Can you work these out from the model? Positions are in its coordinate system, mm. Face numbers are marked on the shaded views. A direction names the side the tool comes from. Coordinates: 2 decimals unless noted, no trailing zeros. Loops run counter-clockwise (first coordinate to the right, second up) from the corner with the lowest first, then second, coordinate; pieces in that order, holes last. Notation, with made-up numbers: M 51.5,84 L 55.5,84 A9 cw 55.5,96 Z; hole C 32.25,67.25 d5. An arc over 180 degrees is marked long. Return JSON: item names as keys, results as strings. Group by question number.
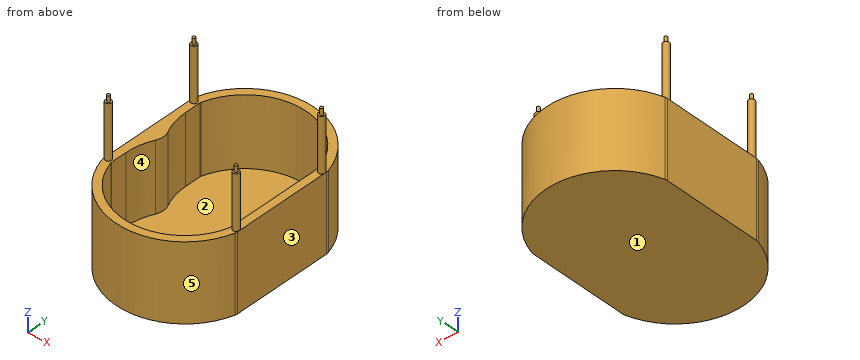
```python
from build123d import *

# Parameters (mm, degrees)
F0_R     = 6
F1_DEPTH = 150
F2_T     = -15
F4_DEPTH = 135
F5_DEPTH = 105
F6_R     = 3
F7_DEPTH = 12


# Not quite as in the source:
# - a feature names something its author has since deleted; it is built from what else it names


with BuildPart() as f1:
    # F0 (on Top) → F1 (new body)
    with BuildSketch(Plane.XY):
        with BuildLine():
            Line((-131, -92.5), (-131, -95.859159479))
            ThreePointArc((-131, -95.859159479), (-130.8132026368, -98.5862460693), (-130.2562998729, -101.2623914012))
            ThreePointArc((-130.2562998729, -101.2623914012), (0, -200), (130.2562998729, -101.2623914012))
            ThreePointArc((130.2562998729, -101.2623914012), (130.8132026368, -98.5862460693), (131, -95.859159479))
            Line((131, -95.859159479), (131, -92.5))
            Line((131, -92.5), (131, 92.5))
            Line((131, 92.5), (131, 95.859159479))
            ThreePointArc((131, 95.859159479), (130.8132026368, 98.5862460693), (130.2562998729, 101.2623914012))
            ThreePointArc((130.2562998729, 101.2623914012), (0, 200), (-130.2562998729, 101.2623914012))
            ThreePointArc((-130.2562998729, 101.2623914012), (-130.8132026368, 98.5862460693), (-131, 95.859159479))
            Line((-131, 95.859159479), (-131, 92.5000001623))
            Line((-131, 92.5000001623), (-131, -92.5))
        make_face()
        with BuildLine():
            ThreePointArc((-119, -92.5), (-125, -98.5), (-131, -92.5))
            ThreePointArc((-131, -92.5), (-125, -86.5), (-119, -92.5))
        make_face(mode=Mode.SUBTRACT)
        with Locations((125, -92.5)):
            Circle(F0_R, mode=Mode.SUBTRACT)
        with BuildLine():
            ThreePointArc((-119, 92.5), (-125.0000000812, 86.5), (-131, 92.5000001623))
            ThreePointArc((-131, 92.5000001623), (-124.9999999188, 98.5), (-119, 92.5))
        make_face(mode=Mode.SUBTRACT)
        with Locations((125, 92.5)):
            Circle(F0_R, mode=Mode.SUBTRACT)
        with BuildLine():
            ThreePointArc((-119, -92.5), (-125, -86.5), (-131, -92.5))
            ThreePointArc((-131, -92.5), (-125, -98.5), (-119, -92.5))
        make_face()
        with BuildLine():
            ThreePointArc((-119, 92.5), (-124.9999999188, 98.5), (-131, 92.5000001623))
            ThreePointArc((-131, 92.5000001623), (-125.0000000812, 86.5), (-119, 92.5))
        make_face()
        with Locations((125, -92.5)):
            Circle(F0_R)
        with Locations((125, 92.5)):
            Circle(F0_R)
    extrude(amount=-F1_DEPTH)

    # F2
    f2_openings = [f1.faces().sort_by_distance(p)[0] for p in [
        (0, 0, 0),
    ]]
    offset(amount=F2_T, openings=f2_openings)

    # F3 (on face) → F4 (join, through all)
    with BuildSketch(Plane.XY):
        with BuildLine():
            ThreePointArc((-103.9827400965, 13.2972029152), (-112.95573879, 38.3122762743), (-116, 64.7130541872))
            Line((-116, 64.7130541872), (-116, -64.7130541872))
            ThreePointArc((-116, -64.7130541872), (-112.95573879, -38.3122762743), (-103.9827400965, -13.2972029152))
            ThreePointArc((-103.9827400965, -13.2972029152), (-100.8748280525, 0), (-103.9827400965, 13.2972029152))
        make_face()
    extrude(amount=-F4_DEPTH)

    # F0 (on Top) → F5 (join)
    with BuildSketch(Plane.XY):
        with Locations((125, -92.5)):
            Circle(F0_R)
        with Locations((125, 92.5)):
            Circle(F0_R)
        with BuildLine():
            ThreePointArc((-119, 92.5), (-124.9999999188, 98.5), (-131, 92.5000001623))
            ThreePointArc((-131, 92.5000001623), (-125.0000000812, 86.5), (-119, 92.5))
        make_face()
        with BuildLine():
            ThreePointArc((-119, -92.5), (-125, -86.5), (-131, -92.5))
            ThreePointArc((-131, -92.5), (-125, -98.5), (-119, -92.5))
        make_face()
    extrude(amount=F5_DEPTH)

    # F6 (on face) → F7 (join)
    with BuildSketch(Plane.XY.offset(105)):
        with Locations((125, -92.5)):
            Circle(F6_R)
        with Locations((-125, -92.5)):
            Circle(F6_R)
        with Locations((125, 92.5)):
            Circle(F6_R)
        with Locations((-125, 92.5)):
            Circle(F6_R)
    extrude(amount=F7_DEPTH)


solid = f1.part
```
1) If we mould it in two halves opening along X, with no side actions, what happens to the marked faces 1, 2 and 3? For each: +X half, -X half, draft (parallel to the pull), parting line (faces both ways), or undercut.
2) For the marked faces 4 and 5, which set-ups out of +Z, -Z, +X, -X, +Y, -Y let a thin tool reach every point of the face, with its end or its side?
3) For pin 1 (12 mm diameter, centred on x = -11, z = -27.5, fed in from +Y); pin 2 (1 mm diameter, centred on x = -75.5, z = -108.5, fed in from -Y); pin 3 (4 mm diameter, centred on x = -87, z = -74.5, fed in from +Y), each with a flat end and sliding along its axis, tell me the tip position at first contact or that it passes through.
4) Suppose I cut it at C-C, the plane x = -33.5. List the corners of the cut face in (y, z) for me.
5) If I drill on line 1 (X direction, y = 78.5, z = -50); line 2 (X direction, y = 97, z = -125); line 3 (Y direction, x = -87, z = -106.5), over which ranges is the centre line in solid material (lowest first)? Write a range as from..to.
6) Suppose I cut it at D-D, the plane z = 54.5. List the corners of the cut face in (x, y) for me.
7) Suppose I cut it at A-A, the plane z = -35. List the corners of the cut face in (x, y) for me.
8) Suppose I cut it at B-B, the plane y = -69.5. List the corners of the cut face in (x, z) for me, then the cut area to 3 significant figures.
Returned:
{
 "1": {"face 1": "draft", "face 2": "undercut", "face 3": "+X half"},
 "2": {"face 4": "+Z", "face 5": "+Z, -Z, -Y"},
 "3": {"pin 1": "stops at y = 199.91", "pin 2": "stops at y = -177.31", "pin 3": "stops at y = 169.96"},
 "4": {"outline": "M -195.79,-150 L 195.79,-150 L 195.79,0 L 180.24,0 L 180.24,-135 L -180.24,-135 L -180.24,0 L -195.79,0 Z"},
 "5": {"line 1": "x = -131..-116, 116..131", "line 2": "x = -130.97..-115.87, 115.87..130.97", "line 3": "y = -168.32..-147.78, 147.78..168.32"},
 "6": {"outline": "C -125,-92.5 d12; C -125,92.5 d12; C 125,-92.5 d12; C 125,92.5 d12"},
 "7": {"outline": "M -131,-95.86 A20 ccw -130.26,-101.26 A135.29 ccw 130.26,-101.26 A20 ccw 131,-95.86 L 131,95.86 A20 ccw 130.26,101.26 A135.29 ccw -130.26,101.26 A20 ccw -131,95.86 Z; hole M -116,-95.86 A5 ccw -115.81,-97.21 A120.29 ccw 115.81,-97.21 A5 ccw 116,-95.86 L 116,95.86 A5 ccw 115.81,97.21 A120.29 ccw -115.81,97.21 A5 ccw -116,95.86 L -116,64.71 A116 ccw -103.98,13.3 A30 cw -103.98,-13.3 A116 ccw -116,-64.71 Z"},
 "8": {"outline": "M -131,-150 L 131,-150 L 131,0 L 116,0 L 116,-135 L -116,-135 L -116,0 L -131,0 Z", "area": "7,980 mm²"}
}
